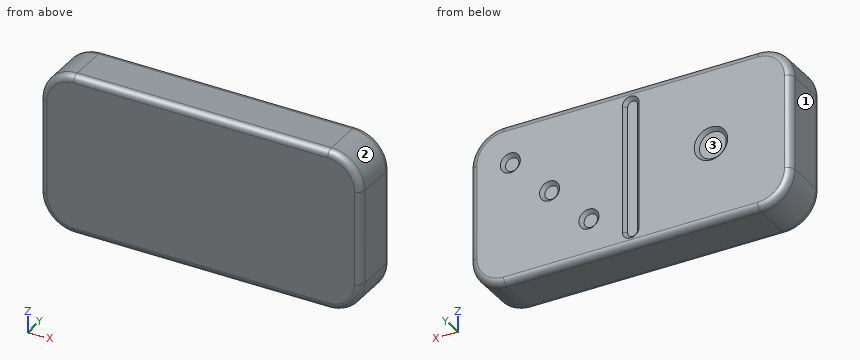
```python
from build123d import *

# Parameters (mm, degrees)
ESQUISSE1_W                = 48
ESQUISSE1_H                = 24
EXTRUSION1_DEPTH           = 7.5
CONG_2_R                   = 5
CONG_5_R                   = 1
CONG_6_R                   = 1
ESQUISSE4_W                = 0.5
ESQUISSE4_H                = 18.982849842
EXTRUSION2_DEPTH           = 0.5
ESQUISSE5_R                = 0.25
EXTRUSION3_DEPTH           = 0.5
CHANFREIN1_SIZE            = 1
ESQUISSE9_R                = 1.5
EXTRUSION6_DEPTH           = 0.5
EXTRUSION6_DRAFT           = -45
EXTRUSION6_PROFILE_2_DEPTH = 0.5
EXTRUSION6_PROFILE_2_DRAFT = -45
EXTRUSION6_PROFILE_3_DEPTH = 0.5
EXTRUSION6_PROFILE_3_DRAFT = -45
ESQUISSE10_R               = 2.5
EXTRUSION8_DEPTH           = 0.5
EXTRUSION8_DRAFT           = -45


with BuildPart() as part:
    # Esquisse1 → Extrusion1 (new body)
    with BuildSketch(Plane(origin=(0, 0, 0), x_dir=(1, 0, 0), z_dir=(0, 1, 0))):
        with Locations((24, 12)):
            Rectangle(ESQUISSE1_W, ESQUISSE1_H)
    extrude(amount=EXTRUSION1_DEPTH)

    # Congé2
    cong_2_edges = [part.edges().sort_by_distance(p)[0] for p in [
        (0, 3.75, -24),
        (48, 3.75, -24),
        (48, 3.75, 0),
        (0, 3.75, 0),
    ]]
    fillet(cong_2_edges, radius=CONG_2_R)

    # Congé5
    cong_5_edges = [part.edges().sort_by_distance(p)[0] for p in [
        (48, 7.5, -12),
        (24, 7.5, 0),
        (0, 7.5, -12),
        (24, 7.5, -24),
        (1.464466094, 7.5, -22.535533906),
        (1.464466094, 7.5, -1.464466094),
        (46.535533906, 7.5, -22.535533906),
        (46.535533906, 7.5, -1.464466094),
    ]]
    fillet(cong_5_edges, radius=CONG_5_R)

    # Congé6
    cong_6_edges = [part.edges().sort_by_distance(p)[0] for p in [
        (48, 0, -12),
        (0, 0, -12),
        (24, 0, -24),
        (24, 0, 0),
        (1.464466094, 0, -22.535533906),
        (1.464466094, 0, -1.464466094),
        (46.535533906, 0, -22.535533906),
        (46.535533906, 0, -1.464466094),
    ]]
    fillet(cong_6_edges, radius=CONG_6_R)

    # Esquisse4 → Extrusion2 (cut)
    with BuildSketch(Plane(origin=(0, 7.5, 0), x_dir=(1, 0, 0), z_dir=(0, 1, 0))):
        with Locations((24, 12)):
            Rectangle(ESQUISSE4_W, ESQUISSE4_H)
    extrude(amount=-EXTRUSION2_DEPTH, mode=Mode.SUBTRACT)

    # Esquisse5 → Extrusion3 (cut)
    with BuildSketch(Plane(origin=(0, 7.5, 0), x_dir=(1, 0, 0), z_dir=(0, 1, 0))):
        with Locations((24, 21.491424921)):
            Circle(ESQUISSE5_R)
        with Locations((24, 2.508575079)):
            Circle(ESQUISSE5_R)
    extrude(amount=-EXTRUSION3_DEPTH, mode=Mode.SUBTRACT)

    # Chanfrein1
    # the kernel refuses this chamfer: 1 mm, written as the material it takes off along each edge
    with BuildSketch(Plane(origin=(24, 7.5, -21.491424921), x_dir=(1, 0, 0), z_dir=(0, 0, 1))) as chanfrein1_piece_1_section:
        Polygon((0.25 + CHANFREIN1_SIZE, 0), (0.25, -CHANFREIN1_SIZE), (0.25, 0), align=None)
    chanfrein1_piece_1 = revolve(axis=Axis((24, 7.5, -21.491424921), (0, 1, 0)), revolution_arc=180, mode=Mode.PRIVATE)
    chanfrein1_piece_1 = split(chanfrein1_piece_1, bisect_by=Plane(origin=(24, 7, -21.964580549), z_dir=(0, 1, 0)), keep=Keep.TOP, mode=Mode.PRIVATE)
    add(chanfrein1_piece_1, mode=Mode.SUBTRACT)
    with BuildSketch(Plane(origin=(24.25, 7.5, -21.491424921), x_dir=(0.9996219169112968, 0.02749587661058651, 0), z_dir=(0, 0, 1))) as chanfrein1_piece_2_section:
        Polygon((CHANFREIN1_SIZE * 0.999621916911, -CHANFREIN1_SIZE * 0.0274958766106), (-CHANFREIN1_SIZE * 0.0274958766106, -CHANFREIN1_SIZE * 0.999621916911), (0, 0), align=None)
    chanfrein1_piece_2 = extrude(amount=18.982849842, mode=Mode.PRIVATE)
    chanfrein1_piece_2 = split(chanfrein1_piece_2, bisect_by=Plane(origin=(24.643401084, 7, -12), z_dir=(0, 1, 0)), keep=Keep.TOP, mode=Mode.PRIVATE)
    add(chanfrein1_piece_2, mode=Mode.SUBTRACT)
    with BuildSketch(Plane(origin=(24, 7.5, -2.508575079), x_dir=(-1, 0, 0), z_dir=(0, 0, -1))) as chanfrein1_piece_3_section:
        Polygon((0.25 + CHANFREIN1_SIZE, 0), (0.25, -CHANFREIN1_SIZE), (0.25, 0), align=None)
    chanfrein1_piece_3 = revolve(axis=Axis((24, 7.5, -2.508575079), (0, 1, 0)), revolution_arc=180, mode=Mode.PRIVATE)
    chanfrein1_piece_3 = split(chanfrein1_piece_3, bisect_by=Plane(origin=(24, 7, -2.035419451), z_dir=(0, 1, 0)), keep=Keep.TOP, mode=Mode.PRIVATE)
    add(chanfrein1_piece_3, mode=Mode.SUBTRACT)
    with BuildSketch(Plane(origin=(23.75, 7.5, -2.508575079), x_dir=(-0.9996219169112968, 0.02749587661058651, 0), z_dir=(0, 0, -1))) as chanfrein1_piece_4_section:
        Polygon((CHANFREIN1_SIZE * 0.999621916911, -CHANFREIN1_SIZE * 0.0274958766106), (-CHANFREIN1_SIZE * 0.0274958766106, -CHANFREIN1_SIZE * 0.999621916911), (0, 0), align=None)
    chanfrein1_piece_4 = extrude(amount=18.982849842, mode=Mode.PRIVATE)
    chanfrein1_piece_4 = split(chanfrein1_piece_4, bisect_by=Plane(origin=(23.356598916, 7, -12), z_dir=(0, 1, 0)), keep=Keep.TOP, mode=Mode.PRIVATE)
    add(chanfrein1_piece_4, mode=Mode.SUBTRACT)


with BuildPart() as extrusion6_tool:
    # Esquisse9 → Extrusion6 (with draft: the straight prism first)
    with BuildSketch(Plane(origin=(0, 7.5, 0), x_dir=(1, 0, 0), z_dir=(0, 1, 0))):
        with Locations((30.25, 18)):
            Circle(ESQUISSE9_R)
    extrude(amount=-EXTRUSION6_DEPTH)
    # Extrusion6: the draft: its side faces are tilted about the plane it starts from
    extrusion6_sides = [extrusion6_tool.faces().sort_by_distance(p)[0] for p in [
        (28.75, 7.25, -18),
    ]]
    draft(extrusion6_sides, Plane(origin=(0, 7.5, 0), x_dir=(1, 0, 0), z_dir=(0, 1, 0)), EXTRUSION6_DRAFT)


with BuildPart() as part_1:
    add(part.part)

    # Extrusion6: cut by extrusion6_tool
    add(extrusion6_tool.part, mode=Mode.SUBTRACT)


with BuildPart() as extrusion6_profile_2_tool:
    # Esquisse9 → Extrusion6 profile 2 (with draft: the straight prism first)
    with BuildSketch(Plane(origin=(0, 7.5, 0), x_dir=(1, 0, 0), z_dir=(0, 1, 0))):
        with Locations((36.125, 12)):
            Circle(ESQUISSE9_R)
    extrude(amount=-EXTRUSION6_PROFILE_2_DEPTH)
    # Extrusion6 profile 2: the draft: its side faces are tilted about the plane it starts from
    extrusion6_profile_2_sides = [extrusion6_profile_2_tool.faces().sort_by_distance(p)[0] for p in [
        (34.625, 7.25, -12),
    ]]
    draft(extrusion6_profile_2_sides, Plane(origin=(0, 7.5, 0), x_dir=(1, 0, 0), z_dir=(0, 1, 0)), EXTRUSION6_PROFILE_2_DRAFT)


with BuildPart() as part_2:
    add(part_1.part)

    # Extrusion6 profile 2: cut by extrusion6_profile_2_tool
    add(extrusion6_profile_2_tool.part, mode=Mode.SUBTRACT)


with BuildPart() as extrusion6_profile_3_tool:
    # Esquisse9 → Extrusion6 profile 3 (with draft: the straight prism first)
    with BuildSketch(Plane(origin=(0, 7.5, 0), x_dir=(1, 0, 0), z_dir=(0, 1, 0))):
        with Locations((42, 6)):
            Circle(ESQUISSE9_R)
    extrude(amount=-EXTRUSION6_PROFILE_3_DEPTH)
    # Extrusion6 profile 3: the draft: its side faces are tilted about the plane it starts from
    extrusion6_profile_3_sides = [extrusion6_profile_3_tool.faces().sort_by_distance(p)[0] for p in [
        (40.5, 7.25, -6),
    ]]
    draft(extrusion6_profile_3_sides, Plane(origin=(0, 7.5, 0), x_dir=(1, 0, 0), z_dir=(0, 1, 0)), EXTRUSION6_PROFILE_3_DRAFT)


with BuildPart() as part_3:
    add(part_2.part)

    # Extrusion6 profile 3: cut by extrusion6_profile_3_tool
    add(extrusion6_profile_3_tool.part, mode=Mode.SUBTRACT)


with BuildPart() as extrusion8_tool:
    # Esquisse10 → Extrusion8 (with draft: the straight prism first)
    with BuildSketch(Plane(origin=(0, 7.5, 0), x_dir=(1, 0, 0), z_dir=(0, 1, 0))):
        with Locations((12, 12)):
            Circle(ESQUISSE10_R)
    extrude(amount=-EXTRUSION8_DEPTH)
    # Extrusion8: the draft: its side faces are tilted about the plane it starts from
    extrusion8_sides = [extrusion8_tool.faces().sort_by_distance(p)[0] for p in [
        (9.5, 7.25, -12),
    ]]
    draft(extrusion8_sides, Plane(origin=(0, 7.5, 0), x_dir=(1, 0, 0), z_dir=(0, 1, 0)), EXTRUSION8_DRAFT)


with BuildPart() as part_4:
    add(part_3.part)

    # Extrusion8: cut by extrusion8_tool
    add(extrusion8_tool.part, mode=Mode.SUBTRACT)


solid = part_4.part
```
Work out the finished part from the listing and answer in its coordinate system (mm). Face numbers are marked on the shaded views. Give positions to 0.01 mm unless a question says otherwise; leave off trailing zeros. Loops run counter-clockwise (first coordinate to the right, second up) from the corner with the lowest first, then second, coordinate; pieces in that order, holes last. Notation, with made-up numbers: (8.25, -24.75) -> (15.25, -24.75) arc R32 cw to (15.25, 9.25) -> close; hole circle Ø3 at (59.5, 44). An arc over 180 degrees is marked (long way). One line per question, with ' | ' between items. Start each with the question number.
1) Straight lines are drawn through the part: L1, parallel to Y at x = 24.5, z = -13.5; L2, parallel to X at y = 0.75, z = -5.25; L3, parallel to Z at x = 41, y = 6.75. For each, find the intervals that lie inside material, in ascending order.
2) Determine the mould class of the marked faces 1, 2 and 3 for opening direction Z: +Z half, -Z half, draft (parallel to the pull), parting line (faces both ways), or undercut.
3) Section A-A, the plane y = 4.25 is taken. Determine the outline of the cut face in (x, z).
4) Section C-C, the plane y = 0.5 is taken. Determine the outline of the cut face in (x, z), then the cut area to 3 significant figures.
5) Each of these flat-tipped pins is pushed along its axis until it touches: pin 1 (2 mm diameter, centred on x = 11.5, z = -12, fed in from +Y); pin 2 (2 mm diameter, centred on x = 30, z = -18, fed in from +Y); pin 3 (1 mm diameter, centred on x = 36.5, z = -12.5, fed in from +Y) (3 decimals). Where does it stop, or does it pass through?
6) Section B-B, the plane x = 12 is taken. Determine the outline of the cut face in (y, z).
Resolved:
1) L1: 0 to 7 | L2: 0.03 to 47.97 | L3: -23.97 to -0.03
2) face 1: draft | face 2: +Z half | face 3: undercut
3) outline: (0, -19) arc R5 ccw to (5, -24) -> (43, -24) arc R5 ccw to (48, -19) -> (48, -5) arc R5 ccw to (43, 0) -> (5, 0) arc R5 ccw to (0, -5) -> close
4) outline: (0.13, -19) arc R4.87 ccw to (5, -23.87) -> (43, -23.87) arc R4.87 ccw to (47.87, -19) -> (47.87, -5) arc R4.87 ccw to (43, -0.13) -> (5, -0.13) arc R4.87 ccw to (0.13, -5) -> close | area: 1,110 mm2
5) pin 1: y = 7 | pin 2: y = 7.25 | pin 3: y = 7.125
6) outline: (0, -23) arc R1 ccw to (1, -24) -> (6.5, -24) arc R1 ccw to (7.5, -23) -> (7.5, -14.5) -> (7, -14) -> (7, -10) -> (7.5, -9.5) -> (7.5, -1) arc R1 ccw to (6.5, 0) -> (1, 0) arc R1 ccw to (0, -1) -> close
